```python
from build123d import *

# Parameters (mm, degrees)
ESQUISSE1_W             = 1.5
ESQUISSE1_H             = 6
ESQUISSE2_R             = 3
BOSS_EXTRU_1_DEPTH      = 1
CHANFREIN1_SIZE         = 1
BOSS_EXTRU_2_START      = 1.5
ESQUISSE3_R             = 3
BOSS_EXTRU_2_DEPTH      = 1.5
CONG_1_R                = 1
ESQUISSE4_R             = 1.25
ENL_V_MAT_EXTRU_1_DEPTH = 8


with BuildPart() as part:
    # Esquisse1 → Révol.-Mince1 (revolve)
    with BuildSketch(Plane.XY, mode=Mode.PRIVATE) as r_vol_mince1_sk:
        with Locations((-0.75, 3)):
            Rectangle(ESQUISSE1_W, ESQUISSE1_H)
    revolve(r_vol_mince1_sk.sketch.rotate(Axis((0, 0, 0), (0, 1, 0)), 270), axis=Axis((0, 0, 0), (0, 1, 0)))

    # Esquisse2 → Boss.-Extru.1 (add)
    with BuildSketch(Plane(origin=(0, 6, 0), x_dir=(1, 0, 0), z_dir=(0, 1, 0))):
        with Locations(Location((0, 0, 0), (0, 0, 270))):
            Circle(ESQUISSE2_R)
    extrude(amount=BOSS_EXTRU_1_DEPTH)

    # Chanfrein1
    chanfrein1_edges = [part.edges().sort_by_distance(p)[0] for p in [
        (0, 7, -3),
    ]]
    chamfer(chanfrein1_edges, length=CHANFREIN1_SIZE - 0.0001)  # a hair under: the kernel refuses the full size

    # Esquisse3 → Boss.-Extru.2 (add)
    with BuildSketch(Plane.XZ.offset(BOSS_EXTRU_2_START)):
        with Locations(Location((0, 0, 0), (0, 0, 270))):
            Circle(ESQUISSE3_R)
    extrude(amount=-BOSS_EXTRU_2_DEPTH)

    # Congé1
    cong_1_edges = [part.edges().sort_by_distance(p)[0] for p in [
        (0, -1.5, 3),
    ]]
    fillet(cong_1_edges, radius=CONG_1_R)

    # Esquisse4 → Enlèv. mat.-Extru.1 (cut)
    with BuildSketch(Plane(origin=(0, -1.5, 0), x_dir=(-1, 0, 0), z_dir=(0, -1, 0))):
        with Locations(Location((0, 0, 0), (0, 0, 90))):
            Circle(ESQUISSE4_R)
    extrude(amount=-ENL_V_MAT_EXTRU_1_DEPTH, mode=Mode.SUBTRACT)


solid = part.part
```
Geometry: final body of the model. Coordinates: model frame, mm. A direction names the side the tool comes from. Coordinates: 2 decimals unless noted, no trailing zeros. Write item = value, one per line.
(1) Access query for faces 1 (the flat face through (0, 7, 0)), 2 (the cylindrical face through (-0.45, 3.04, -1.43)). Directions: +Z, -Z, +X, -X, +Y, -Y. A direction counts if a zero-diameter tool reaches every point of the face in a straight line with its end or side. Return the directions, or none.
Solved:
face_1 = +Z, -Z, +X, -X, +Y
face_2 = none
(2) Pull-direction query (Y, two-part tool) for faces 3 (the flat face through (0, 6.5, 0)), 4 (the cylindrical face through (-1.22, 2.44, 0.27)), 5 (the flat face through (-1.3, 6, 1.3)); classes: pulls with the +Y half, pulls with the -Y half, needs draft (parallel to the pull), parting line crosses it, or undercut.
Solved:
face_3 = pulls with the -Y half
face_4 = needs draft
face_5 = undercut
(3) Pin query (flat end, axial travel): pin 1 Ø1 at (y, z) = (1.5, -1) entering from -X; pin 2 Ø2 at (x, z) = (0, 0) entering from -Y. Return the tip coordinate at first contact, or that it passes through.
Solved:
pin_1 = -1.41
pin_2 = 6.5
(4) Line query: line 1 (X direction, y = 1.75, z = 0); line 2 (Y direction, x = -1.5, z = 1); line 3 (X direction, y = 4.5, z = 0.95). Output: solid intervals per line, ascending.
Solved:
line_1 = -1.5 to -1.25, 1.25 to 1.5
line_2 = -1.5 to 0, 6 to 7
line_3 = -1.16 to -0.81, 0.81 to 1.16
